```python
from build123d import *

# Parameters (mm, degrees)
F1_DEPTH  = 127
F0_W      = 50.8
F0_H      = 12.7
F2_DEPTH  = 63.5
F3_W      = 38.1
F3_H      = 12.7
F4_DEPTH  = 50.8
F5_R      = 3.81
F6_DEPTH  = 50.8
F7_R      = 3.81
F8_DEPTH  = 50.8
F9_R      = 3.81
F10_DEPTH = 50.8


with BuildPart() as f1:
    # F0 (on Right) → F1 (new body)
    with BuildSketch(Plane.YZ):
        Polygon((37.902087, -44.522293), (37.902087, 107.877707), (-9.190773, 88.827707), (-9.190773, -38.172293), (37.902087, -57.222293), align=None)
    extrude(amount=F1_DEPTH)

    # F0 (on Right) → F2 (join)
    with BuildSketch(Plane.YZ):
        with Locations((63.302087, -50.872293)):
            Rectangle(F0_W, F0_H)
    extrude(amount=F2_DEPTH)

    # F3 (on face) → F4 (join)
    with BuildSketch(Plane(origin=(0, 37.902087, 0), x_dir=(-1, 0, 0), z_dir=(0, 1, 0))):
        with Locations((-107.95, -50.872293)):
            Rectangle(F3_W, F3_H)
        with Locations((-107.95, 101.527707)):
            Rectangle(F3_W, F3_H)
    extrude(amount=F4_DEPTH)

    # F5 (on face) → F6 (cut)
    with BuildSketch(Plane(origin=(0, 88.702087, 0), x_dir=(-1, 0, 0), z_dir=(0, 1, 0))):
        with Locations((-96.52, 101.527707)):
            Circle(F5_R)
        with Locations((-119.38, 101.527707)):
            Circle(F5_R)
    extrude(amount=-F6_DEPTH, mode=Mode.SUBTRACT)

    # F7 (on face) → F8 (cut)
    with BuildSketch(Plane(origin=(0, 88.702087, 0), x_dir=(-1, 0, 0), z_dir=(0, 1, 0))):
        with Locations((-96.52, -50.872293)):
            Circle(F7_R)
        with Locations((-119.38, -50.872293)):
            Circle(F7_R)
    extrude(amount=-F8_DEPTH, mode=Mode.SUBTRACT)

    # F9 (on face) → F10 (cut)
    with BuildSketch(Plane(origin=(0, 88.702087, 0), x_dir=(-1, 0, 0), z_dir=(0, 1, 0))):
        with Locations((-55.88, -50.872293)):
            Circle(F9_R)
        with Locations((-7.62, -50.872293)):
            Circle(F9_R)
    extrude(amount=-F10_DEPTH, mode=Mode.SUBTRACT)


solid = f1.part
```
Part model, mm, in its own coordinate system. A direction names the side the tool comes from. Round coordinates to 2 decimals unless told otherwise and drop trailing zeros. Loops run counter-clockwise (first coordinate to the right, second up) from the corner with the lowest first, then second, coordinate; pieces in that order, holes last. Notation, with made-up numbers: (-1, 16) -> (45, 16) arc R6 ccw to (45, 25) -> close; hole circle Ø11 at (5.25, -17.5). An arc over 180 degrees is marked (long way). Use one line per item in the form item = value. Start each with the question number.
Item 1: Band-saw the part on D-D (x = 55.88). List the corners of the cut face in (y, z).
Item 2: Band-saw the part on C-C (z = -2). List the corners of the cut face in (x, y), plus the area to 3 significant figures.
Item 3: Drop flat-ended pins along their axis: pin 1 Ø1.5 at (x, z) = (73, -31.5) entering from +Y; pin 2 Ø1 at (x, y) = (31, 45.5) entering from +Z; pin 3 Ø10 at (x, z) = (119.38, -50.87) entering from -Y; pin 4 Ø10 at (y, z) = (57, -38) entering from -X. Give the stop position or say it passes through.
Item 4: Tool access for faces 4 (the flat face through (108, 63, 95.178)), 5 (the flat face through (31, 63, -44.522)), 6 (the cylindrical face through (100.326, 63.658, 101.695)): list every direction of +Z, -Z, +X, -X, +Y, -Y with a clear straight run to the whole face (end or side of a thin tool).
Item 5: Drill centre lines: line 1 along Z through (x, y) = (119.38, 58.5); line 2 along Z through (x, y) = (7.62, 52); line 3 along X through (y, z) = (40, 100). Where is each one in solid material? Low to high.
Item 6: Band-saw the part on B-B (x = 96.52). List the corners of the cut face in (y, z).
Item 7: Band-saw the part on A-A (y = 73.5). Give the number of separate pieces and of enclosed holes in the cut face, plus the area to 3 significant figures.
Item 8: Two-plate mould, pull along X, no slides. Class faces 1 (the flat face through (88.9, 63, -51)), 2 (the flat face through (62.61, 14.69, 98.49)), 3 (the flat face through (0, 17, 8)): released by +X, released by -X, zero draft, split by the parting line, or undercut.
Data:
q1.outline = (-9.19, -38.17) -> (37.9, -57.22) -> (88.7, -57.22) -> (88.7, -54.68) -> (37.9, -54.68) -> (37.9, -47.06) -> (88.7, -47.06) -> (88.7, -44.52) -> (37.9, -44.52) -> (37.9, 107.88) -> (-9.19, 88.83) -> close
q2.outline = (0, -9.19) -> (127, -9.19) -> (127, 37.9) -> (0, 37.9) -> close
q2.area = 5,980 mm^2
q3.pin_1 = 37.9
q3.pin_2 = -44.52
q3.pin_3 = 9.84
q3.pin_4 = through
q4.face_4 = +X, -X, +Y
q4.face_5 = +Z, +X, -X, +Y
q4.face_6 = +Y
q5.line_1 = -57.22 to -54.68, -47.06 to -44.52, 95.18 to 97.72, 105.34 to 107.88
q5.line_2 = -57.22 to -54.68, -47.06 to -44.52
q5.line_3 = 88.9 to 93.03, 100.01 to 115.89, 122.87 to 127
q6.outline = (-9.19, -38.17) -> (37.9, -57.22) -> (88.7, -57.22) -> (88.7, -54.68) -> (37.9, -54.68) -> (37.9, -47.06) -> (88.7, -47.06) -> (88.7, -44.52) -> (37.9, -44.52) -> (37.9, 95.18) -> (88.7, 95.18) -> (88.7, 97.72) -> (37.9, 97.72) -> (37.9, 105.34) -> (88.7, 105.34) -> (88.7, 107.88) -> (37.9, 107.88) -> (-9.19, 88.83) -> close
q7.separate_pieces = 3
q7.enclosed_holes = 6
q7.area = 1,500 mm^2
q8.face_1 = undercut
q8.face_2 = zero draft
q8.face_3 = released by -X
